Input: part model. Units: mm. Frame: model coordinates. A direction names the side the tool comes from. Give positions to 0.01 mm unless a question says otherwise; leave off trailing zeros. Order: outer loops, then holes, each group sorted by start corner. A loop starts at its lowest first (then second) coordinate and runs counter-clockwise, first axis right, second up. Notation, with made-up numbers: (-16.5, 82) - (31.5, 82) arc R32 ccw to (31.5, 112) - close; hole circle Ø7 at (21, 63). An arc over 180 degrees is marked (long way). Answer in a Markdown table with one row per item. Add a question column.
1. Section query A-A on y = 49. Return loops of the section in (x, z), and give its area (3 significant figures).
2. Contact query for flat-ended pins moving along their axis: pin 1 (15 mm diameter, centred on x = 107.5, z = 29.5, fed in from -Y); pin 2 (9 mm diameter, centred on x = 48.5, y = 115, fed in from -Z); pin 3 (12 mm diameter, centred on x = 73.5, y = 77.5, fed in from +Z). Output: stop coordinate, or through.
3. Mould query, pull axis Y, two halves, no side actions, for faces 1 (the face through (55.95, 24.1, 4.93)), 2 (the face through (110, 70, 74.5)), 3 (the face through (51, 40.372, 5)). Classes: released by +Y, released by -Y, zero draft, split by the parting line, or undercut.
4. Ray query, line 1 (Y direction, x = 88.5, z = 29); line 2 (X direction, y = 10.5, z = 63); line 3 (Z direction, x = 92, y = 35.5). Return the intervals inside material, ascending. Write a range as [from, to].
5. Section query B-B on x = 86.5. Return loops of the section in (y, z), and give its area (3 significant figures).
6. Access query for faces 4 (the face through (86.25, 4.57, 4.93)), 5 (the face through (85, 119.962, 37)), 6 (the face through (51, 116, 4)), 7 (the face through (112.007, -8, 39)). Directions: +Z, -Z, +X, -X, +Y, -Y. A direction counts if a zero-diameter tool reaches every point of the face in a straight line with its end or side. Return the directions, or none.
7. Section query C-C on z = 46.5. Return loops of the section in (x, y).
```python
from build123d import *

# Parameters (mm, degrees)
EXTRUDE_1_DEPTH     = 10
EXTRUDE_2_DEPTH     = 64.5
SKETCH_4_W          = 3.8
SKETCH_4_H          = 69.5
EXTRUDE_4_DEPTH     = 1
EXTRUDE_5_DEPTH     = 69.5
EXTRUDE_6_DEPTH     = 70.5
FILLET_1_R          = 2
SKETCH_7_W          = 70.5
SKETCH_7_H          = 3.8
EXTRUDE_7_DEPTH     = 6
CUT_EXTRUDE_1_REACH = 185.071


with BuildPart() as part:
    # 草圖1 → 填料-伸長1 (new body)
    with BuildSketch(Plane.XY):
        Polygon((116.20678675, 119.962196633), (116.20678675, -4.797282637), (104.20678675, -4.797282637), (104.20678675, -5.797282637), (69.565770598, 14.202717363), (54.456814697, 40.372196633), (54.456814697, 119.962196633), align=None)
        Polygon((54.456814697, 40.372196633), (46.554726499, 40.372196633), (65.614726499, 7.35930824), (69.565770598, 14.202717363), align=None)
    extrude(amount=EXTRUDE_1_DEPTH)

    # 草圖2 → 填料-伸長2 (add)
    with BuildSketch(Plane.XY.offset(10)):
        Polygon((108.20678675, -4.797282637), (116.20678675, -4.797282637), (116.20678675, 119.962196633), (54.456814697, 119.962196633), (54.456814697, 111.962196633), (108.20678675, 111.962196633), align=None)
    extrude(amount=EXTRUDE_2_DEPTH)

    # 草圖4 → 填料-伸長4 (add)
    with BuildSketch(Plane.XZ.offset(4.797282637)):
        with Locations((110.10678675, 39.75)):
            Rectangle(SKETCH_4_W, SKETCH_4_H)
    extrude(amount=EXTRUDE_4_DEPTH)

    # 草圖5 → 填料-伸長5 (add)
    with BuildSketch(Plane(origin=(0, 0, 5), x_dir=(-1, 0, 0), z_dir=(0, 0, -1))):
        Polygon((-108.20678675, -5.797282637), (-108.20678675, -8.106683714), (-112.00678675, -10.300614737), (-112.00678675, -5.797282637), align=None)
    extrude(amount=-EXTRUDE_5_DEPTH)

    # 草圖6 → 填料-伸長6 (add)
    with BuildSketch(Plane.XY.offset(74.5)):
        Polygon((50.992713082, 113.962196633), (54.456814697, 111.962196633), (54.456814697, 116.350058678), (52.892713082, 117.253093167), align=None)
    extrude(amount=-EXTRUDE_6_DEPTH)

    # 圓角1
    fillet_1_edges = [part.edges().sort_by_distance(p)[0] for p in [
        (85.331800723, 119.962196633, 0),
        (116.20678675, 57.582456998, 0),
        (116.20678675, 119.962196633, 37.25),
        (116.20678675, 57.582456998, 74.5),
        (85.331800723, 119.962196633, 74.5),
    ]]
    fillet(fillet_1_edges, radius=FILLET_1_R)

    # 草圖7 → 填料-伸長7 (add)
    with BuildSketch(Plane(origin=(-11.102543866, 6.41005669, 0), x_dir=(0, 0, 1), z_dir=(-0.8660254037844396, 0.4999999999999985, 0))):
        with Locations((39.25, 126.090513896)):
            Rectangle(SKETCH_7_W, SKETCH_7_H)
    extrude(amount=EXTRUDE_7_DEPTH)

    # 草圖8 → 除料-伸長1 (cut, up to next)
    with BuildSketch(Plane(origin=(0, 0, 0), x_dir=(-1, 0, 0), z_dir=(0, 0, -1)), mode=Mode.PRIVATE) as cut_extrude_1_sk1:
        Polygon((-104.20678675, -4.797282637), (-102.474735942, -4.797282637), (-104.20678675, -5.797282637), align=None)
    cut_extrude_1_tool1 = extrude(cut_extrude_1_sk1.sketch, amount=-CUT_EXTRUDE_1_REACH, mode=Mode.PRIVATE) & part.part
    add(cut_extrude_1_tool1.solids().sort_by_distance((103.629436, -5.130616, 0))[0], mode=Mode.SUBTRACT)


solid = part.part
```
Answer:
| question | item | result |
|---|---|---|
| 1 | outline | (54.46, 0) - (114.21, 0) arc R2 ccw to (116.21, 2) - (116.21, 72.5) arc R2 ccw to (114.21, 74.5) - (108.21, 74.5) - (108.21, 10) - (54.46, 10) - close |
| 1 | area | 1,130 mm² |
| 2 | pin 1 | stops at y = -10.3 |
| 2 | pin 2 | stops at z = 4 |
| 2 | pin 3 | stops at z = 10 |
| 3 | face 1 | released by -Y |
| 3 | face 2 | zero draft |
| 3 | face 3 | undercut |
| 4 | line 1 | y = [111.96, 119.96] |
| 4 | line 2 | x = [108.21, 116.21] |
| 4 | line 3 | z = [0, 10] |
| 5 | outline | (4.43, 0) - (117.96, 0) arc R2 ccw to (119.96, 2) - (119.96, 72.5) arc R2 ccw to (117.96, 74.5) - (111.96, 74.5) - (111.96, 10) - (4.43, 10) - close |
| 5 | area | 1,670 mm² |
| 6 | face 4 | +Z, -Z, -Y |
| 6 | face 5 | +Z, -Z, +X, +Y |
| 6 | face 6 | -Z, -X, +Y |
| 6 | face 7 | +Z, -Z, +X, -Y |
| 7 | outline | (45.8, 116.96) - (54.46, 111.96) - (108.21, 111.96) - (108.21, -8.11) - (112.01, -10.3) - (112.01, -4.8) - (116.21, -4.8) - (116.21, 117.96) arc R2 ccw to (114.21, 119.96) - (54.46, 119.96) - (54.46, 116.35) - (47.7, 120.25) - close |
